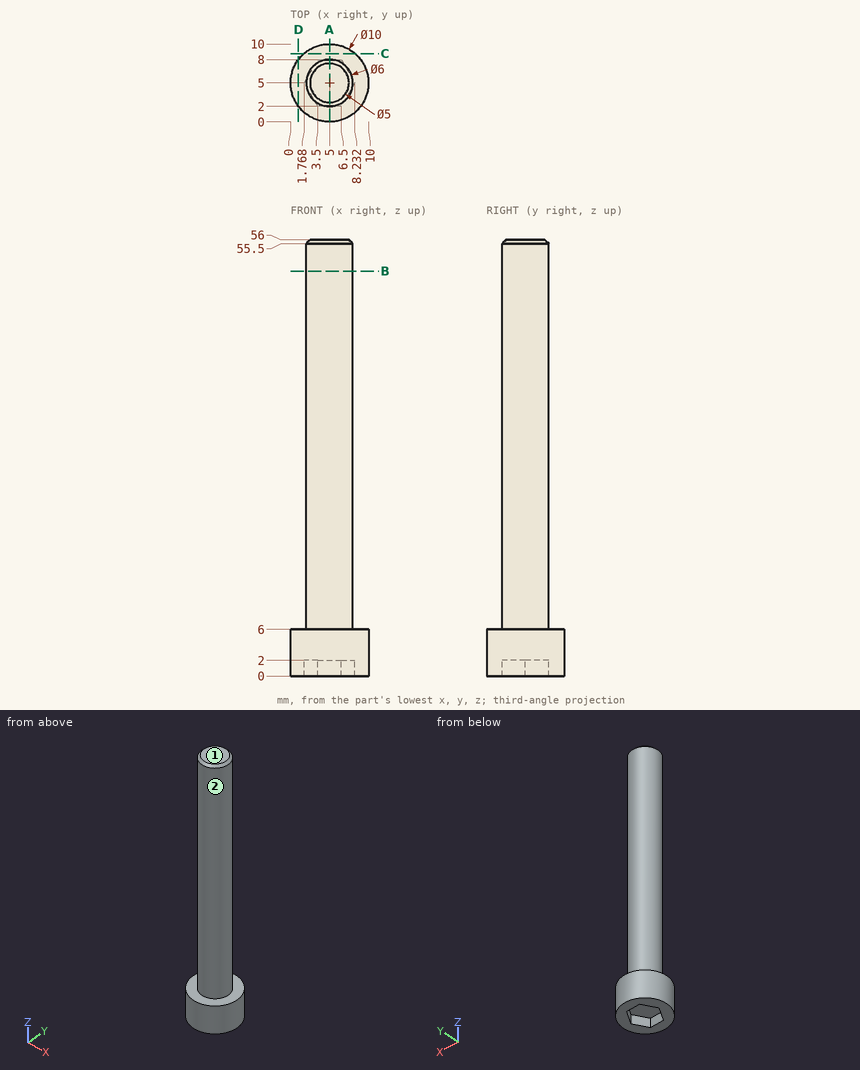
Geometry check sheet. Reference: drawing and pictorial views, mm from the part's lowest x, y, z. Give positions to 0.01 mm unless a question says otherwise; leave off trailing zeros. Loops run counter-clockwise (first coordinate to the right, second up) from the corner with the lowest first, then second, coordinate; pieces in that order, holes last. Notation, with made-up numbers: M 88,-12 L 130,-12 A11 cw 130,6 Z; hole C 63,-17.5 d5. An arc over 180 degrees is marked long. One line per question, with ' | ' between items.
Item 1: Section check B-B, the plane z = 52. Record the cut outline in (x, y).
Completed:
outline: C 5,5 d6
Item 2: Section check C-C, the plane y = 8.75. Record the cut outline in (x, z).
Completed:
outline: M 1.69,0 L 8.31,0 L 8.31,6 L 1.69,6 Z
Item 3: Section check A-A, the plane x = 5. Record the cut outline in (y, z), plus the area to 3 significant figures.
Completed:
outline: M 0,0 L 2,0 L 2,2 L 8,2 L 8,0 L 10,0 L 10,6 L 8,6 L 8,55.5 L 7.5,56 L 2.5,56 L 2,55.5 L 2,6 L 0,6 Z | area: 348 mm^2
Item 4: Section check D-D, the plane x = 1. Record the cut outline in (y, z), plus the area to 3 significant figures.
Completed:
outline: M 2,0 L 8,0 L 8,6 L 2,6 Z | area: 36.0 mm^2
Item 5: Thickness scan on line 1 (Y direction, x = 4.75, z = 13); line 2 (Z direction, x = 3, y = 3.5); line 3 (Z direction, x = 6.25, y = 1). Record the ranges inside material, lowest first. Write a range as [from, to].
Completed:
line 1: y = [2.01, 7.99] | line 2: z = [2, 56] | line 3: z = [0, 6]
Item 6: Draft check along Z on the marked faces 1 and 2. Enter one of: +Z half, -Z half, draft (parallel to the pull), parting line (faces both ways), or undercut.
Completed:
face 1: +Z half | face 2: draft
Item 7: Depth check by flat-ended pin: P1, Ø2, axis at x = 5.5, z = 45.5, coming from the +Y side; P2, Ø1, axis at x = 8, z = 40, coming from the +Y side; P3, Ø4, axis at x = 4.5, z = 27, coming from the -Y side. Enter the tip coordinate at first touch or a pass-through.
Completed:
P1: stops at y = 8 | P2: stops at y = 6.66 | P3: stops at y = 2
